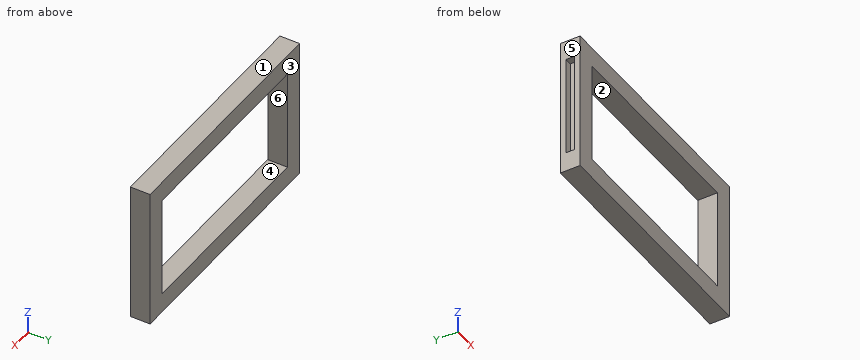
from build123d import *

# Parameters (mm, degrees)
F0_W          = 860
F0_H          = 500
F0_W_2        = 720
F0_H_2        = 360
F1_DEPTH      = 70
F3_W          = 30
F3_H          = 360
F4_DEPTH      = 25
F4_DEPTH_BACK = 25
F5_SCALE      = 0.4


# Not quite as in the source:
# - a feature names something its author has since deleted; it is built from what else it names


with BuildPart() as f1:
    # F0 (on Front) → F1 (new body)
    with BuildSketch(Plane.XZ):
        with Locations((-61.0144731402, -34.6215157021)):
            Rectangle(F0_W, F0_H)
        with Locations((-61.0144731402, -34.6215157021)):
            Rectangle(F0_W_2, F0_H_2, mode=Mode.SUBTRACT)
    extrude(amount=F1_DEPTH)

    # F3 (on face) → F4 (cut, two sides)
    with BuildSketch(Plane(origin=(-491.0144731402, 0, 0), x_dir=(0, -1, 0), z_dir=(-1, 0, 0))) as f4_sk:
        with Locations((35, -34.6215157021)):
            Rectangle(F3_W, F3_H)
    extrude(amount=F4_DEPTH, mode=Mode.SUBTRACT)
    extrude(f4_sk.sketch, amount=-F4_DEPTH_BACK, mode=Mode.SUBTRACT)


with BuildPart() as f1_1:
    # F5: moved
    add(f1.part.scale(F5_SCALE).moved(Location((-294.6086838841, 0, -170.7729094213))))


solid = f1_1.part
Model file for the job. Use its own axes, mm. Face numbers are marked on the shaded views. A direction names the side the tool comes from. Give positions to 0.01 mm unless a question says otherwise; leave off trailing zeros. Loops run counter-clockwise (first coordinate to the right, second up) from the corner with the lowest first, then second, coordinate; pieces in that order, holes last.
1) Flat gauge pins, fed straight in: pin 1 Ø5 at (x, z) = (-483.5, -187.5) entering from +Y; pin 2 Ø9.5 at (y, z) = (-14.5, -186) entering from -X. Where does each tip first touch, or does it go through?
2) Pull direction Z, two halves, no side cores. Call the marked faces 1, 2, 3 and 4: +Z half, -Z half, draft (parallel to the pull), parting line (faces both ways), or undercut.
3) Saw through at A-A (x = -184). Write the cut outline in (y, z), plus the area to 3 significant figures.
4) Tool access for the marked faces 5 and 6: list every direction of +Z, -Z, +X, -X, +Y, -Y with a clear straight run to the whole face (end or side of a thin tool).
5) Saw through at C-C (y = -4). Write the cut outline in (x, z), plus the area to 3 significant figures.
6) Wall check: line 1 (Z direction, x = -425, y = -13); line 2 (X direction, y = -13.5, z = -150); line 3 (X direction, y = -22.25, z = -184.5). Give the ranges that are in metal, low to high.
7) Saw through at B-B (z = -118.5). Write the cut outline in (x, y).
Answer block:
1. pin 1: stops at y = 0
1. pin 2: stops at x = -481.01
2. face 1: +Z half
2. face 2: undercut
2. face 3: draft
2. face 4: undercut
3. outline: (-28, -284.62) - (0, -284.62) - (0, -256.62) - (-28, -256.62) - close; (-28, -112.62) - (0, -112.62) - (0, -84.62) - (-28, -84.62) - close
3. area: 1,570 mm2
4. face 5: +Z, -Z, -X, +Y, -Y
4. face 6: +Y, -Y
5. outline: (-491.01, -284.62) - (-147.01, -284.62) - (-147.01, -84.62) - (-491.01, -84.62) - close; hole (-463.01, -256.62) - (-175.01, -256.62) - (-175.01, -112.62) - (-463.01, -112.62) - close
5. area: 27,300 mm2
6. line 1: z = -284.62 to -256.62, -112.62 to -84.62
6. line 2: x = -481.01 to -463.01, -175.01 to -147.01
6. line 3: x = -491.01 to -463.01, -175.01 to -147.01
7. outline: (-491.01, -28) - (-463.01, -28) - (-463.01, 0) - (-491.01, 0) - (-491.01, -8) - (-481.01, -8) - (-481.01, -20) - (-491.01, -20) - close; (-175.01, -28) - (-147.01, -28) - (-147.01, 0) - (-175.01, 0) - close
